Build history of the part. All positions in model axes, mm. Coordinates: 2 decimals unless noted, no trailing zeros. Order: outer loops, then holes, each group sorted by start corner. A loop starts at its lowest first (then second) coordinate and runs counter-clockwise, first axis right, second up. Notation, with made-up numbers: (36.5, 32.25) -> (61.5, 32.25) arc R24 cw to (61.5, 68.25) -> close; hole circle Ø11 at (29.5, 76.25). An arc over 180 degrees is marked (long way). Write each question's results on one line, items separated by ' | '.
Autodesk Inventor part; units mm, degrees
ref_plane "YZ Plane" through (0, 0, 0) normal (1, 0, 0) x (0, 1, 0)
ref_plane "XZ Plane" through (0, 0, 0) normal (0, 1, 0) x (-1, 0, 0)
ref_plane "XY Plane" through (0, 0, 0) normal (0, 0, 1) x (1, 0, 0)
sketch "Sketch1" plane through (0, 0, 0) normal (0, 1, 0) x (-1, 0, 0)
  circle A0 centre (0, 0) radius 2.0955
  circle A1 centre (-25.4, 0) radius 2.0955
  arc A2 (0, -6.35) -> (0, 6.35) centre (0, 0) ccw
  arc A3 (-25.4, 6.35) -> (-25.4, -6.35) centre (-25.4, 0) ccw
  line L0 (0, 6.35) -> (-25.4, 6.35)
  line L1 (-25.4, -6.35) -> (0, -6.35)
  dimension "d0" = 4.191
  dimension "d1" = 4.191
  dimension "d2" = 12.7
  dimension "d3" = 12.7
extrude "Extrusion1" add sketch "Sketch1" along normal blind 1.5875
properties part number "Gear Shield" material "Acetal Resin, White"
Item 1: Pull direction X, two halves, no side cores. Call faces 1 (the cylindrical face through (31.75, 0.78, -0.14)), 2 (the cylindrical face through (-6.35, 0.78, 0.14)), 3 (the cylindrical face through (-2, 0.78, -0.63)), 4 (the flat face through (13, 1.588, 0)): released by +X, released by -X, zero draft, split by the parting line, or undercut.
Answer:
face 1: released by +X | face 2: released by -X | face 3: undercut | face 4: zero draft
Item 2: Pin check, flat tip, straight feed: pin 1 (4 mm diameter, centred on x = 25.4, z = 0, fed in from -Y). Stop position of the tip, or through.
Answer:
pin 1: passes through
Item 3: Slice it at C-C, the plane x = -3.5. List the corners of the cut face in (y, z).
Answer:
outline: (0, -5.3) -> (1.59, -5.3) -> (1.59, 5.3) -> (0, 5.3) -> close
Item 4: Slice it at B-B, the plane y = 0.8. List the corners of the cut face in (x, z), and give its area (3 significant figures).
Answer:
outline: (0, -6.35) -> (25.4, -6.35) arc R6.35 ccw to (25.4, 6.35) -> (0, 6.35) arc R6.35 ccw to start; hole circle Ø4.19 at (0, 0); hole circle Ø4.19 at (25.4, 0) | area: 422 mm^2
Item 5: Slice it at A-A, the plane z = 0. List the corners of the cut face in (x, y), and give its area (3 significant figures).
Answer:
outline: (-6.35, 0) -> (-2.1, 0) -> (-2.1, 1.59) -> (-6.35, 1.59) -> close; (2.1, 0) -> (23.3, 0) -> (23.3, 1.59) -> (2.1, 1.59) -> close; (27.5, 0) -> (31.75, 0) -> (31.75, 1.59) -> (27.5, 1.59) -> close | area: 47.2 mm^2
Item 6: Drill centre lines: line 1 (Z direction, x = 0, y = 0.35); line 2 (X direction, y = 0.65, z = -1.25). Where is each one in solid material? Low to high. Write a range as from..to.
Answer:
line 1: z = -6.35..-2.1, 2.1..6.35 | line 2: x = -6.23..-1.68, 1.68..23.72, 27.08..31.63
Item 7: Slice it at D-D, the plane z = -4.5. List the corners of the cut face in (x, y), and give its area (3 significant figures).
Answer:
outline: (-4.48, 0) -> (29.88, 0) -> (29.88, 1.59) -> (-4.48, 1.59) -> close | area: 54.5 mm^2
